Input: part model. Units: mm. Frame: model coordinates. Face numbers are marked on the shaded views. A direction names the side the tool comes from. Coordinates: 2 decimals unless noted, no trailing zeros. Write each loop counter-clockwise with the first axis right and the second up, starting at its lowest first coordinate (ties: lowest second). Pieces come first, ordered by that corner, then holes. Notation, with made-up numbers: (59, -35) - (80, -35) arc R30 cw to (80, -6) - close; hole circle Ø2 at (-3, 49.5). An arc over 180 degrees is marked (long way). One line per question, with ' | ' between items. Start each with the question number.
1) Draft query along X for the marked faces 3, 4, 5 and 6. Return one class per face: released by +X, released by -X, zero draft, split by the parting line, or undercut.
2) Section query B-B on z = 11.5. Return loops of the section in (x, y), and give its area (3 significant figures).
3) Section query A-A on x = 20. Return loops of the section in (y, z), and give its area (3 significant figures).
4) First-contact query: P1, Ø7, axis at x = -20, y = 0, coming from the -Z side; P2, Ø3, axis at x = -20, y = 0, coming from the -Z side. Flat tips, straight axial feed; report the tip coordinate or a pass-through.
5) Section query D-D on y = 0. Return loops of the section in (x, z), and give its area (3 significant figures).
6) Section query C-C on y = 7.25. Return loops of the section in (x, z), and give its area (3 significant figures).
7) Reachability of the marked faces 1 and 2 from +Z, -Z, +X, -X, +Y, -Y: full face, straight path, thin tool, end or side. Return the list, or none.
8) Line query: line 1 (Y direction, x = 20, z = 2.1); line 2 (X direction, y = 0, z = 6); line 3 (Y direction, x = 20, z = 7.5). Output: solid intervals per line, ascending.
```python
from build123d import *

# Parameters (mm, degrees)
SKETCH2_W           = 50
SKETCH2_H           = 20
SKETCH2_R           = 1.7
BOSS_EXTRUDE1_DEPTH = 8
BOSS_EXTRUDE2_DEPTH = 20
SKETCH6_R           = 3.75
CUT_EXTRUDE1_DEPTH  = 4
SKETCH7_R           = 1.7
CUT_EXTRUDE2_DEPTH  = 13.8


with BuildPart() as part:
    # Sketch2 → Boss-Extrude1 (new body)
    with BuildSketch(Plane.XY):
        Rectangle(SKETCH2_W, SKETCH2_H)
        with Locations((-20, 0)):
            Circle(SKETCH2_R, mode=Mode.SUBTRACT)
        with Locations((20, 0)):
            Circle(SKETCH2_R, mode=Mode.SUBTRACT)
    extrude(amount=BOSS_EXTRUDE1_DEPTH)

    # Sketch5 → Boss-Extrude2 (add)
    with BuildSketch(Plane.XZ.offset(10)):
        with BuildLine():
            Line((-25, 8), (-25, 12.8))
            Line((-25, 12.8), (-10.1, 12.8))
            Line((-10.1, 12.8), (-10.1, 8))
            Line((-10.1, 8), (10.1, 8))
            Line((10.1, 8), (10.1, 12.8))
            Line((10.1, 12.8), (25, 12.8))
            Line((25, 12.8), (25, 8))
            ThreePointArc((25, 8), (0, 0), (-25, 8))
        make_face()
    extrude(amount=-BOSS_EXTRUDE2_DEPTH)

    # Sketch6 → Cut-Extrude1 (cut)
    with BuildSketch(Plane(origin=(0, 0, 0), x_dir=(-1, 0, 0), z_dir=(0, 0, -1))):
        with Locations((20, 0)):
            Circle(SKETCH6_R)
        with Locations((-20, 0)):
            Circle(SKETCH6_R)
    extrude(amount=-CUT_EXTRUDE1_DEPTH, mode=Mode.SUBTRACT)

    # Sketch7 → Cut-Extrude2 (cut, through all)
    with BuildSketch(Plane(origin=(0, 0, 0), x_dir=(-1, 0, 0), z_dir=(0, 0, -1))):
        with Locations((20, 0)):
            Circle(SKETCH7_R)
        with Locations((-20, 0)):
            Circle(SKETCH7_R)
    extrude(amount=-CUT_EXTRUDE2_DEPTH, mode=Mode.SUBTRACT)


solid = part.part
```
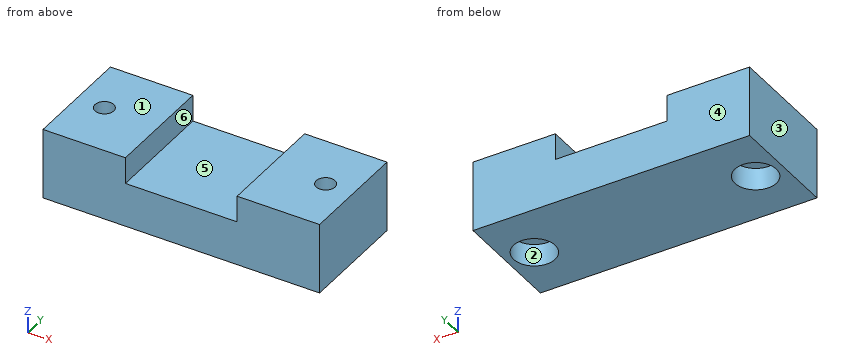
Answer key:
1) face 3: released by -X | face 4: zero draft | face 5: undercut | face 6: undercut
2) outline: (-25, -10) - (-10.1, -10) - (-10.1, 10) - (-25, 10) - close; (10.1, -10) - (25, -10) - (25, 10) - (10.1, 10) - close; hole circle Ø3.4 at (-20, 0); hole circle Ø3.4 at (20, 0) | area: 578 mm²
3) outline: (-10, 0) - (-3.75, 0) - (-3.75, 4) - (-1.7, 4) - (-1.7, 12.8) - (-10, 12.8) - close; (1.7, 4) - (3.75, 4) - (3.75, 0) - (10, 0) - (10, 12.8) - (1.7, 12.8) - close | area: 196 mm²
4) P1: z = 4 | P2: through
5) outline: (-25, 0) - (-23.75, 0) - (-23.75, 4) - (-21.7, 4) - (-21.7, 12.8) - (-25, 12.8) - close; (-18.3, 4) - (-16.25, 4) - (-16.25, 0) - (16.25, 0) - (16.25, 4) - (18.3, 4) - (18.3, 12.8) - (10.1, 12.8) - (10.1, 8) - (-10.1, 8) - (-10.1, 12.8) - (-18.3, 12.8) - close; (21.7, 4) - (23.75, 4) - (23.75, 0) - (25, 0) - (25, 12.8) - (21.7, 12.8) - close | area: 423 mm²
6) outline: (-25, 0) - (25, 0) - (25, 12.8) - (10.1, 12.8) - (10.1, 8) - (-10.1, 8) - (-10.1, 12.8) - (-25, 12.8) - close | area: 543 mm²
7) face 1: +Z, +X, -X, +Y, -Y | face 2: -Z
8) line 1: -10 to -3.75, 3.75 to 10 | line 2: -25 to -21.7, -18.3 to 18.3, 21.7 to 25 | line 3: -10 to -1.7, 1.7 to 10
